Could you check a few things on this model? Use its own coordinates, in mm. A direction names the side the tool comes from. Round coordinates to 2 decimals unless told otherwise and drop trailing zeros. Loops run counter-clockwise (first coordinate to the right, second up) from the corner with the lowest first, then second, coordinate; pieces in that order, holes last.
Autodesk Inventor part; units mm, degrees
ref_plane "YZ Plane" through (0, 0, 0) normal (1, 0, 0) x (0, 1, 0)
ref_plane "XZ Plane" through (0, 0, 0) normal (0, 1, 0) x (-1, 0, 0)
ref_plane "XY Plane" through (0, 0, 0) normal (0, 0, 1) x (1, 0, 0)
sketch "Sketch2" plane through (0, 0, 0) normal (0, 0, 1) x (1, 0, 0)
  line L0 (-17, 28) -> (0, 28)
  line L1 (0, 28) -> (0, 17)
  line L2 (0, 7) -> (0, 0)
  line L3 (0, 0) -> (-17, 0)
  line L4 (-17, 0) -> (-17, 7)
  line L5 (-17, 28) -> (-17, 17)
  line L6 (-17, 17) -> (-17, 7)
  line L7 (0, 17) -> (0, 7)
  dimension "d0" = 17
  dimension "d1" = 28
extrude "Extrusion1" add sketch "Sketch2" along normal blind 5
sketch "Sketch4" plane through (0, 0, 0) normal (0, 0, -1) x (-1, 0, 0)
  line L0 (17, 28) -> (0, 28)
  line L1 (0, 28) -> (0, 0)
  line L2 (0, 0) -> (17, 0)
  line L3 (17, 0) -> (17, 28)
  line L4 (0, 28) -> (17, 28)
  line L5 (11.5, 24) -> (11.5, 4)
  line L6 (11.5, 4) -> (5.5, 4)
  line L7 (5.5, 4) -> (5.5, 24)
  line L8 (5.5, 24) -> (11.5, 24)
  dimension "d15" = 6
  dimension "d17" = 5.5
  dimension "d30" = 20
  dimension "d31" = 4
extrude "Extrusion3" cut sketch "Sketch4" against normal blind 1.5 contours L5 L6 L7 L8
sketch "Sketch5" plane through (0, 0, 5) normal (0, 0, 1) x (1, 0, 0)
  line L0 (0, 28) -> (-17, 28)
  line L1 (-17, 28) -> (-17, 0)
  line L2 (-17, 0) -> (0, 0)
  line L3 (0, 0) -> (0, 28)
  line L4 (-21, 17) -> (4, 7)
  line L5 (-21.4753, 7) -> (4, 17)
  circle A0 centre (-8.6177, 12.0471) radius 5
  dimension "d20" = 10
  dimension "d21" = 12.0471
extrude "Extrusion4" cut sketch "Sketch5" against normal through all contours A0 L4 L5 | L5 L4 A0 | L4 L5 A0 | A0 L5 L4
sketch "Sketch6" plane through (0, 0, 5) normal (0, 0, 1) x (1, 0, 0)
  circle A0 centre (-8.6177, 12.0471) radius 5
  line L0 (0, 28) -> (-17, 28)
  line L1 (-17, 28) -> (-17, 0)
  line L2 (-17, 0) -> (0, 0)
  line L3 (0, 0) -> (0, 28)
  circle A1 centre (-12.5, 26) radius 1.35
  dimension "d24" = 2.7
  dimension "d25" = 4.5
  dimension "d26" = 2
extrude "Extrusion5" cut sketch "Sketch6" against normal through all contours A1
sketch "Sketch7" plane through (0, 0, 5) normal (0, 0, 1) x (1, 0, 0)
  line L0 (0, 0) -> (0, 28)
  line L1 (-17, 0) -> (0, 0)
  circle A0 centre (-4.5, 5) radius 1.35
  point P0 (0, 7)
  dimension "d32" = 2.7
  dimension "d33" = 4.5
  dimension "d34" = 5
extrude "Extrusion6" cut sketch "Sketch7" against normal through all
sketch "Sketch8" plane through (0, 0, 0) normal (1, 0, 0) x (0, 0, -1)
  circle A0 centre (-2, 12) radius 1.6
  line L0 (-5, 0) -> (-5, 28)
  line L1 (0, 0) -> (-5, 0)
  point P0 (0, -7)
  dimension "d37" = 3.2
  dimension "d41" = 12
  dimension "d49" = 3
extrude "Extrusion8" cut sketch "Sketch8" against normal through all
sketch "Sketch9" plane through (0, 0, 5) normal (0, 0, 1) x (1, 0, 0)
  circle A0 centre (-4.5, 5) radius 1.35
  circle A1 centre (-12.5, 26) radius 1.35
  circle A2 centre (-8.6177, 12.0471) radius 5
  line L0 (0, 28) -> (-17, 28)
  line L1 (-17, 28) -> (-17, 0)
  line L2 (-17, 0) -> (0, 0)
  line L3 (0, 0) -> (0, 28)
  line L4 (-17, 0) -> (-16.5, 0)
  line L5 (-16.5, 0) -> (-16.5, 28)
  line L6 (-16.5, 28) -> (-17, 28)
  line L7 (-17, 28) -> (-17, 0)
  line L8 (0, 0) -> (-0.5, 0)
  line L9 (-0.5, 0) -> (-0.5, 28)
  line L10 (-0.5, 28) -> (0, 28)
  line L11 (0, 28) -> (0, 0)
  dimension "d47" = 0.5
  dimension "d48" = 0.5
extrude "Extrusion9" cut sketch "Sketch9" against normal through all contours L3 L2 L9 L0 | L5 L2 L1 L0
properties part number "tapa0.2"
Item 1: For faces 5 (the cylindrical face through (-3.212, 5.406, 2.535)), 6 (the flat face through (-5.5, 20, 1)), which set-ups out of +Z, -Z, +X, -X, +Y, -Y let a thin tool reach every point of the face, with its end or its side?
Results list:
face 5: +Z, -Z
face 6: -Z
Item 2: Will these pins go through, and if not, where does the flat tip stop? pin 1 (1.6 mm diameter, centred on x = -4.5, y = 5, fed in from +Z); pin 2 (3 mm diameter, centred on x = -8, y = 20.5, fed in from -Z).
Results list:
pin 1: passes through
pin 2: stops at z = 1.5
Item 3: If we section it at C-C, the plane x = -8.5: Please give me the cut outline in (y, z), then the cut area to 3 significant figures.
Results list:
outline: (0, 0) - (4, 0) - (4, 1.5) - (7.05, 1.5) - (7.05, 5) - (0, 5) - close; (17.05, 1.5) - (24, 1.5) - (24, 0) - (28, 0) - (28, 5) - (17.05, 5) - close
area: 75.0 mm2
Item 4: If we section it at B-B, the plane z = 3.15: Please give me the cut outline in (x, y).
Results list:
outline: (-16.5, 0) - (-0.5, 0) - (-0.5, 10.89) - (-3.75, 10.89) arc R5 cw to (-13.48, 10.89) - (-16.5, 10.89) - close; (-16.5, 13.11) - (-13.5, 13.11) arc R5 cw to (-3.73, 13.11) - (-0.5, 13.11) - (-0.5, 28) - (-16.5, 28) - close; hole circle Ø2.7 at (-12.5, 26); hole circle Ø2.7 at (-4.5, 5)
Item 5: If we section it at D-D, the plane y = 13: Please give me the cut outline in (x, z).
Results list:
outline: (-16.5, 0) - (-13.53, 0) - (-13.53, 0.75) - (-16.5, 0.75) - close; (-16.5, 3.25) - (-13.53, 3.25) - (-13.53, 5) - (-16.5, 5) - close; (-3.71, 0) - (-0.5, 0) - (-0.5, 0.75) - (-3.71, 0.75) - close; (-3.71, 3.25) - (-0.5, 3.25) - (-0.5, 5) - (-3.71, 5) - close
Item 6: We'd pull the mould along Y, two halves only. Please class faces 1 (the flat face through (-8, 0, 2)), 2 (the flat face through (-12, 17, 0)), 3 (the flat face through (-11.5, 6, 1)), 4 (the flat face through (-9, 4, 1)): released by +Y, released by -Y, zero draft, split by the parting line, or undercut.
Results list:
face 1: released by -Y
face 2: zero draft
face 3: undercut
face 4: undercut
Item 7: If I drill on line 1 along Z through (x, y) = (-14.55, 12); line 2 along Y through (x, z) = (-14.3, 2); line 3 along Y through (x, z) = (-6, 1.35), over which ranges is the centre line in solid material (lowest first)?
Results list:
line 1: z = 0 to 0.4, 3.6 to 5
line 2: y = 0 to 10.4, 13.6 to 28
line 3: y = 0 to 4, 24 to 28
Item 8: If we section it at A-A, the plane y = 26: Please give me the cut outline in (x, z), then the cut area to 3 significant figures.
Results list:
outline: (-16.5, 0) - (-13.85, 0) - (-13.85, 5) - (-16.5, 5) - close; (-11.15, 0) - (-0.5, 0) - (-0.5, 5) - (-11.15, 5) - close
area: 66.5 mm2
